Autodesk Fusion 360 part; units mm, degrees
sketch "3D-printed conduit outline" plane through (0, 0, 0) normal (0, 1, 0) x (1, 0, 0)
  line L0 (0, 0) -> (16, 0)
  line L1 (16, 0) -> (16, -14)
  line L2 (16, -14) -> (0, -14)
  line L3 (0, -14) -> (0, 0)
  line L4 (2, -14) -> (14, -14)
  line L5 (14, -14) -> (14, -2)
  line L6 (14, -2) -> (2, -2)
  line L7 (2, -2) -> (2, -14)
  dimension "d8" = 14
  dimension "d9" = 16
  dimension "d10" = 2
  dimension "d11" = 2
  dimension "d12" = 2
extrude "Extrude1" add sketch "3D-printed conduit outline" along normal blind 182 contours L0 L1 L2 L3 L5 L6 L7
sketch "Magnet holders" plane through (0, 0, 14) normal (0, 0, 1) x (-1, 0, 0)
  line L0 (0, 0) -> (-2, 0)
  line L1 (-2, 0) -> (-2, -182)
  line L2 (-2, -182) -> (0, -182)
  line L3 (0, -182) -> (0, 0)
  line L4 (-14, 0) -> (-16, 0)
  line L5 (-16, 0) -> (-16, -182)
  line L6 (-16, -182) -> (-14, -182)
  line L7 (-14, -182) -> (-14, 0)
  circle A0 centre (-2.5, -2.5) radius 2.5
  circle A1 centre (-2.5, -2.5) radius 1.75
  line L8 (-14, 0) -> (-2, 0)
  line L9 (0, 0) -> (-2.5, 0)
  line L10 (-2.5, 0) -> (-2.5, -5)
  line L11 (-2.5, -5) -> (0, -5)
  line L12 (0, -5) -> (0, 0)
  circle A2 centre (-13.5, -2.5) radius 2.5
  circle A3 centre (-13.5, -2.5) radius 1.75
  line L13 (-16, 0) -> (-13.5, 0)
  line L14 (-13.5, 0) -> (-13.5, -5)
  line L15 (-13.5, -5) -> (-16, -5)
  line L16 (-16, -5) -> (-16, 0)
  circle A4 centre (-2.5, -61.5) radius 1.75
  circle A5 centre (-2.5, -61.5) radius 2.5
  line L17 (-2.5, -59) -> (-2.5, -64)
  line L18 (-2.5, -64) -> (0, -64)
  line L19 (0, -64) -> (0, -59)
  line L20 (0, -59) -> (-2.5, -59)
  circle A6 centre (-13.5, -61.5) radius 1.75
  circle A7 centre (-13.5, -61.5) radius 2.5
  line L21 (-13.5, -59) -> (-13.5, -64)
  line L22 (-13.5, -64) -> (-16, -64)
  line L23 (-16, -64) -> (-16, -59)
  line L24 (-16, -59) -> (-13.5, -59)
  circle A8 centre (-2.5, -120.5) radius 1.75
  circle A9 centre (-2.5, -120.5) radius 2.5
  line L25 (-2.5, -118) -> (-2.5, -123)
  line L26 (-2.5, -123) -> (0, -123)
  line L27 (0, -123) -> (0, -118)
  line L28 (0, -118) -> (-2.5, -118)
  circle A10 centre (-13.5, -120.5) radius 1.75
  circle A11 centre (-13.5, -120.5) radius 2.5
  line L29 (-13.5, -118) -> (-13.5, -123)
  line L30 (-13.5, -123) -> (-16, -123)
  line L31 (-16, -123) -> (-16, -118)
  line L32 (-16, -118) -> (-13.5, -118)
  circle A12 centre (-2.5, -179.5) radius 1.75
  circle A13 centre (-2.5, -179.5) radius 2.5
  line L33 (-2.5, -177) -> (-2.5, -182)
  line L34 (-2.5, -182) -> (0, -182)
  line L35 (0, -182) -> (0, -177)
  line L36 (0, -177) -> (-2.5, -177)
  circle A14 centre (-13.5, -179.5) radius 1.75
  circle A15 centre (-13.5, -179.5) radius 2.5
  line L37 (-13.5, -177) -> (-13.5, -182)
  line L38 (-13.5, -182) -> (-16, -182)
  line L39 (-16, -182) -> (-16, -177)
  line L40 (-16, -177) -> (-13.5, -177)
  dimension "d15" = 5
  dimension "d16" = 3.5
  dimension "d17" = 5
  dimension "d18" = 3.5
  dimension "d21" = 0
  dimension "d22" = -177
extrude "Extrude2" add sketch "Magnet holders" against normal blind 3 contours A2 A3 L14 | L7 A2 A3 L14 | L7 L8 A2 L13 | L1 A0 L8 L9 | L1 A0 A1 L10 | A0 A1 L10 | L1 A0 A1 L10 | L1 A0 L11 | L1 A1 L10 | A1 L10 | L7 A3 L14 | A3 L14 | L1 A5 L20 | L7 A2 L15 | L7 A2 A3 L14 | L1 A4 A5 L17 | L1 A4 A5 L17 | L1 A5 L18 | A4 A5 L17 | L1 A4 L17 | A4 L17 | L7 A7 L24 | L1 A9 L28 | L7 A6 A7 L21 | A6 A7 L21 | L1 A8 A9 L25 | L1 A8 A9 L25 | L1 A9 L26 | A8 A9 L25 | L7 A6 L21 | A6 L21 | L7 A7 L22 | L7 A6 A7 L21 | L1 A8 L25 | A8 L25 | L1 A13 L36 | L7 A11 L32 | L1 A12 A13 L33 | L1 A12 A13 L33 | L1 A13 L34 | A12 A13 L33 | L7 A10 A11 L29 | L7 A11 L30 | L7 A10 A11 L29 | A10 A11 L29 | L1 A12 L33 | A12 L33 | L7 A10 L29 | A10 L29 | L7 A15 L40 | L7 A14 A15 L37 | L7 A15 L38 | L7 A14 A15 L37 | A14 A15 L37 | L7 A14 L37 | A14 L37
extrude "Extrude3" cut sketch "Magnet holders" against normal blind 1 contours L1 A1 | L1 A1 L10 | A1 L10 | L7 A3 L14 | A3 L14 | L7 A3 | L1 A4 | L1 A4 L17 | A4 L17 | L7 A6 L21 | L7 A6 | A6 L21 | L1 A8 | L1 A8 L25 | A8 L25 | L1 A12 | L1 A12 L33 | A12 L33 | L7 A10 L29 | L7 A10 | A10 L29 | L7 A14 L37 | L7 A14 | A14 L37
chamfer "Chamfer1" distance 1 angle 45 2 edges at (2, 91, 2) (14, 91, 2)
chamfer "Chamfer2" distance 2.9999 angle 45 8 edges at (2, 2.5, 11) (2, 61.5, 11) (2, 120.5, 11) (2, 179.5, 11) (14, 2.5, 11) (14, 61.5, 11) (14, 120.5, 11) (14, 179.5, 11)
equation "conduit_length = 182.00 mm"
equation "conduit_width = 16 mm"
equation "conduit_height = 16 mm"
equation "conduit_wall_thickness = 2 mm"
equation "magnet_diameter = 3 mm"
equation "magnet_height = 1 mm"
equation "d8 = conduit_height - conduit_wall_thickness"
equation "d9 = conduit_width"
equation "d10 = conduit_wall_thickness"
equation "d11 = conduit_wall_thickness"
equation "d12 = conduit_wall_thickness"
equation "d13 = conduit_length"
equation "d15 = magnet_diameter + 2 mm"
equation "d16 = magnet_diameter + 0.5 mm"
equation "d17 = magnet_diameter + 2 mm"
equation "d18 = magnet_diameter + 0.5 mm"
equation "d22 = -conduit_length + ( magnet_diameter + 2 mm )"
equation "d23 = -( magnet_height + 2 mm )"
Check sheet for the modelled part. Datum: model origin and axes. Units: mm. A direction names the side the tool comes from. Give positions to 0.01 mm unless a question says otherwise; leave off trailing zeros. Loops run counter-clockwise (first coordinate to the right, second up) from the corner with the lowest first, then second, coordinate; pieces in that order, holes last. Notation, with made-up numbers: M 39,-16 L 64,-16 A22 ccw 64,-2 Z; hole C 89.5,10.25 d3. An arc over 180 degrees is marked long. Use a Markdown table: item, result. Add a question column.
Q1. Scan lines: line 1 along X through (y, z) = (179.5, 13.65); line 2 along X through (y, z) = (50, 4); line 3 along Z through (x, y) = (4, 8). Record each from-to range of solid material in increasing order. Write a range as [from, to].
Q2. Sectioned sample at B-B, the plane y = 80. Record the cut outline in (x, z).
Q3. Mould release check, pull along Y, two halves, no side actions. Record for faces 1 (the flat face through (3, 61, 9)), 2 (the cylindrical face through (12.69, 181.05, 13.51)), 3 (the cylindrical face through (12.6, 119, 13.5)): pulls with the +Y half, pulls with the -Y half, needs draft (parallel to the pull), parting line crosses it, or undercut.
Q4. Sectioned sample at C-C, the plane x = 7. Record the cut outline in (y, z), then the cut area to 3 significant figures.
Q5. Sectioned sample at A-A, the plane z = 5.5. Record the cut outline in (x, y), then the cut area to 3 significant figures.
Q6. Go/stop test with flat-tipped pins: pin 1 (3 mm diameter, centred on x = 13.5, y = 179.5, fed in from +Z); pin 2 (5 mm diameter, centred on x = 6, z = 11, fed in from +Y). Record where each tip stops, or that it passes through.
Q7. Tool access check on faces 4 (the flat face through (3, 120, 9)), 5 (the flat face through (16, 90, 7)), 6 (the flat face through (3, 2, 13)). Record the directions out of +Z, -Z, +X, -X, +Y, -Y that give a thin tool (end or side, any length) a straight path to the whole face; none if there is none.
Verdict:
| question | item | result |
|---|---|---|
| 1 | line 1 | [0, 0.75], [4.25, 5], [11, 11.75], [15.25, 16] |
| 1 | line 2 | [0, 2], [14, 16] |
| 1 | line 3 | [0, 2] |
| 2 | outline | M 0,0 L 16,0 L 16,14 L 14,14 L 14,3 L 13,2 L 3,2 L 2,3 L 2,14 L 0,14 Z |
| 3 | face 1 | needs draft |
| 3 | face 2 | undercut |
| 3 | face 3 | undercut |
| 4 | outline | M 0,0 L 182,0 L 182,2 L 0,2 Z |
| 4 | area | 364 mm^2 |
| 5 | outline | M 0,0 L 2,0 L 2,182 L 0,182 Z; M 14,0 L 16,0 L 16,182 L 14,182 Z |
| 5 | area | 728 mm^2 |
| 6 | pin 1 | z = 13 |
| 6 | pin 2 | y = 181.79 |
| 7 | face 4 | +Y, -Y |
| 7 | face 5 | +Z, -Z, +X, +Y, -Y |
| 7 | face 6 | +Z |
